```python
from build123d import *

# Parameters (mm, degrees)
SKETCH1_R           = 3.5
SKETCH1_R_2         = 1.5
BOSS_EXTRUDE1_DEPTH = 9
SKETCH2_R           = 6
SKETCH2_R_2         = 1.5
BOSS_EXTRUDE2_DEPTH = 3
SKETCH3_R           = 5
SKETCH3_R_2         = 1.5
BOSS_EXTRUDE3_DEPTH = 3
FILLET2_R           = 1
SKETCH4_R           = 10
SKETCH4_R_2         = 1.5
BOSS_EXTRUDE4_DEPTH = 3
SKETCH5_R           = 10
SKETCH5_R_2         = 1.5
BOSS_EXTRUDE5_DEPTH = 3


with BuildPart() as part:
    # Sketch1 → Boss-Extrude1 (new body)
    with BuildSketch(Plane(origin=(0, 0, 0), x_dir=(1, 0, 0), z_dir=(0, 1, 0))):
        Circle(SKETCH1_R)
        Circle(SKETCH1_R_2, mode=Mode.SUBTRACT)
    extrude(amount=BOSS_EXTRUDE1_DEPTH)

    # Sketch2 → Boss-Extrude2 (add)
    with BuildSketch(Plane(origin=(0, 9, 0), x_dir=(1, 0, 0), z_dir=(0, 1, 0))):
        Circle(SKETCH2_R)
        Circle(SKETCH2_R_2, mode=Mode.SUBTRACT)
    extrude(amount=-BOSS_EXTRUDE2_DEPTH)

    # Sketch3 → Boss-Extrude3 (add)
    with BuildSketch(Plane.XZ):
        Circle(SKETCH3_R)
        Circle(SKETCH3_R_2, mode=Mode.SUBTRACT)
    extrude(amount=-BOSS_EXTRUDE3_DEPTH)

    # Fillet2
    fillet2_edges = [part.edges().sort_by_distance(p)[0] for p in [
        (-3.5, 6, 0),
        (-3.5, 3, 0),
    ]]
    fillet(fillet2_edges, radius=FILLET2_R)

    # Sketch4 → Boss-Extrude4 (add)
    with BuildSketch(Plane.XZ):
        Circle(SKETCH4_R)
        Circle(SKETCH4_R_2, mode=Mode.SUBTRACT)
    extrude(amount=-BOSS_EXTRUDE4_DEPTH)

    # Sketch5 → Boss-Extrude5 (add)
    with BuildSketch(Plane(origin=(0, 9, 0), x_dir=(1, 0, 0), z_dir=(0, 1, 0))):
        Circle(SKETCH5_R)
        Circle(SKETCH5_R_2, mode=Mode.SUBTRACT)
    extrude(amount=-BOSS_EXTRUDE5_DEPTH)


solid = part.part
```
Check sheet for the modelled part. Datum: model origin and axes. Units: mm. A direction names the side the tool comes from. Coordinates: 2 decimals unless noted, no trailing zeros. Write each loop counter-clockwise with the first axis right and the second up, starting at its lowest first coordinate (ties: lowest second). Pieces come first, ordered by that corner, then holes. Notation, with made-up numbers: (11.25, 77) -> (49.25, 77) arc R22 ccw to (49.25, 94) -> close; hole circle Ø2 at (-33.75, 13.5). An arc over 180 degrees is marked (long way). Use a Markdown table: item, result.
1. Sectioned sample at B-B (x = 8). Enter the section's corners in (y, z).
Reported:
| item | result |
|---|---|
| outline | (0, -6) -> (3, -6) -> (3, 6) -> (0, 6) -> close; (6, -6) -> (9, -6) -> (9, 6) -> (6, 6) -> close |
2. Sectioned sample at A-A (z = 0). Enter the section's corners in (x, y), plus the area to 3 significant figures.
Reported:
| item | result |
|---|---|
| outline | (-10, 0) -> (-1.5, 0) -> (-1.5, 9) -> (-10, 9) -> (-10, 6) -> (-4.5, 6) arc R1 cw to (-3.5, 5) -> (-3.5, 4) arc R1 cw to (-4.5, 3) -> (-10, 3) -> close; (1.5, 0) -> (10, 0) -> (10, 3) -> (4.5, 3) arc R1 cw to (3.5, 4) -> (3.5, 5) arc R1 cw to (4.5, 6) -> (10, 6) -> (10, 9) -> (1.5, 9) -> close |
| area | 115 mm2 |
3. Sectioned sample at D-D (y = 0.75). Enter the section's corners in (x, z), plus the area to 3 significant figures.
Reported:
| item | result |
|---|---|
| outline | circle Ø20 at (0, 0); hole circle Ø3 at (0, 0) |
| area | 307 mm2 |
4. Go/stop test with flat-tipped pins: pin 1 Ø2 at (y, z) = (6, 8) entering from +X; pin 2 Ø2.5 at (x, z) = (0, 0) entering from +Y (3 decimals); pin 3 Ø8 at (x, z) = (4.5, -7.5) entering from -Y. Record where each tip stops, or that it passes through.
Reported:
| item | result |
|---|---|
| pin 1 | stops at x = 7.14 |
| pin 2 | passes through |
| pin 3 | stops at y = 0 |
5. Sectioned sample at C-C (x = 0). Enter the section's corners in (y, z), plus the area to 3 significant figures.
Reported:
| item | result |
|---|---|
| outline | (0, -10) -> (3, -10) -> (3, -4.5) arc R1 cw to (4, -3.5) -> (5, -3.5) arc R1 cw to (6, -4.5) -> (6, -10) -> (9, -10) -> (9, -1.5) -> (0, -1.5) -> close; (0, 1.5) -> (9, 1.5) -> (9, 10) -> (6, 10) -> (6, 4.5) arc R1 cw to (5, 3.5) -> (4, 3.5) arc R1 cw to (3, 4.5) -> (3, 10) -> (0, 10) -> close |
| area | 115 mm2 |
6. Tool access check on faces 4 (the flat face through (4.3, 3, -2.1)), 5 (the cylindrical face through (-1.5, 4.44, -0.07)). Record the directions out of +Z, -Z, +X, -X, +Y, -Y that give a thin tool (end or side, any length) a straight path to the whole face; none if there is none.
Reported:
| item | result |
|---|---|
| face 4 | none |
| face 5 | +Y, -Y |
7. Release check for a two-part mould opening along Y. For faces 1 (the flat face through (2, 0, 0)), 2 (the cylindrical face through (-2.17, 1.48, -9.76)), 3 (the cylindrical face through (3.233, 4.493, 1.341)) record: pulls with the +Y half, pulls with the -Y half, needs draft (parallel to the pull), parting line crosses it, or undercut.
Reported:
| item | result |
|---|---|
| face 1 | pulls with the -Y half |
| face 2 | needs draft |
| face 3 | undercut |
8. Scan lines: line 1 along Y through (x, z) = (-6.25, 6); line 2 along X through (y, z) = (6.5, 0); line 3 along Z through (x, y) = (0, 4.75). Record each from-to range of solid material in increasing order.
Reported:
| item | result |
|---|---|
| line 1 | y = 0 to 3, 6 to 9 |
| line 2 | x = -10 to -1.5, 1.5 to 10 |
| line 3 | z = -3.5 to -1.5, 1.5 to 3.5 |
